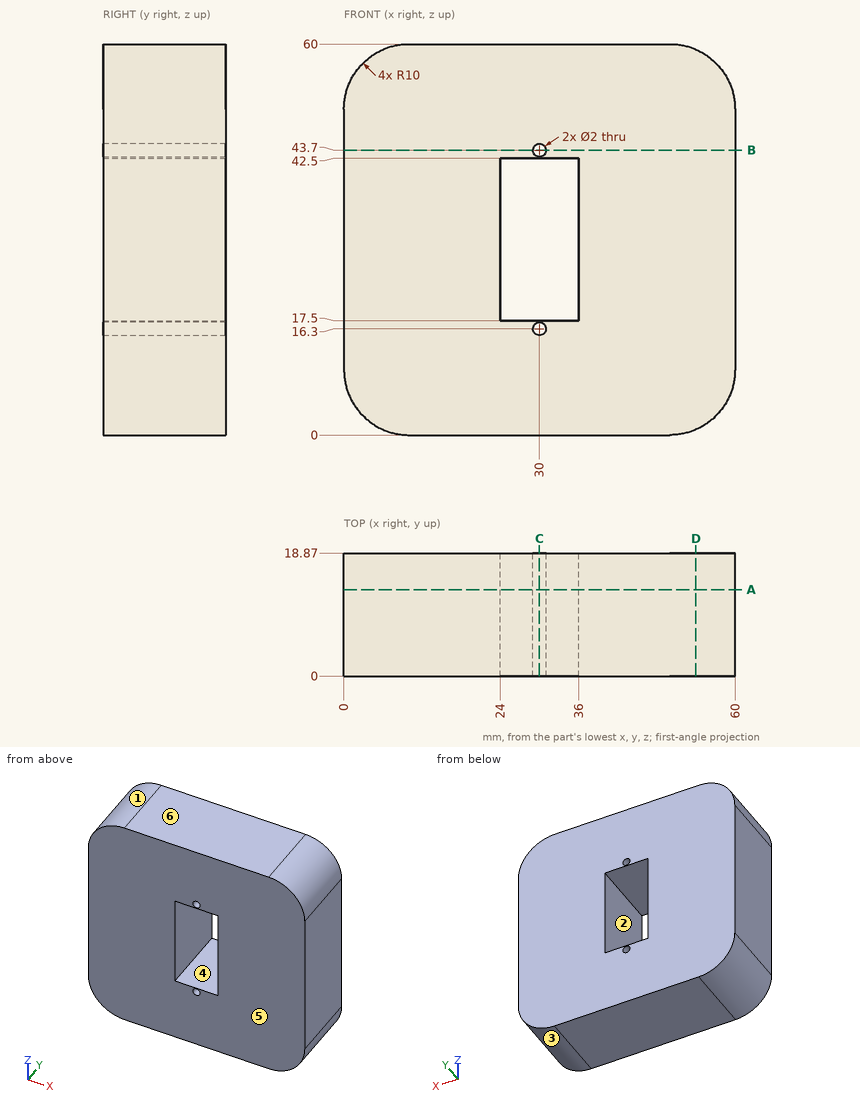
Here's the drawing with two shaded views (mm, measured from the low corner). I have some questions. A direction names the side the tool comes from. Coordinates: 2 decimals unless noted, no trailing zeros. Order: outer loops, then holes, each group sorted by start corner. A loop starts at its lowest first (then second) coordinate and runs counter-clockwise, first axis right, second up.
Item 1: If we section it at D-D on x = 54: List the corners of the cut face in (y, z) for me, plus the area to 3 significant figures.
Result sheet:
outline: (0, 0.83) - (18.87, 0.83) - (18.87, 59.17) - (0, 59.17) - close
area: 1,100 mm2
Item 2: If we section it at B-B on z = 43.7: List the corners of the cut face in (x, y) for me.
Result sheet:
outline: (0, 0) - (29, 0) - (29, 18.87) - (0, 18.87) - close; (31, 0) - (60, 0) - (60, 18.87) - (31, 18.87) - close
Item 3: I need wall thicknesses on line 1 (X direction, y = 5, z = 16.3); line 2 (Z direction, x = 35, y = 11.5); line 3 (X direction, y = 5.75, z = 23). Which ranges of each line are inside material? Lowest first, please.
Result sheet:
line 1: x = 0 to 29, 31 to 60
line 2: z = 0 to 17.5, 42.5 to 60
line 3: x = 0 to 24, 36 to 60
Item 4: If we section it at A-A on y = 13.25: List the corners of the cut face in (x, z) for me.
Result sheet:
outline: (0, 10) arc R10 ccw to (10, 0) - (50, 0) arc R10 ccw to (60, 10) - (60, 50) arc R10 ccw to (50, 60) - (10, 60) arc R10 ccw to (0, 50) - close; hole (24, 17.5) - (36, 17.5) - (36, 42.5) - (24, 42.5) - close; hole circle Ø2 at (30, 16.3); hole circle Ø2 at (30, 43.7)
Item 5: For the marked faces 1 and 2, which set-ups out of +Z, -Z, +X, -X, +Y, -Y let a thin tool reach every point of the face, with its end or its side?
Result sheet:
face 1: +Z, -X, +Y, -Y
face 2: +Y, -Y
Item 6: If we mould it in two halves opening along Z, with no side actions, what happens to the marked faces 3, 4, 5 and 6? For each: +Z half, -Z half, draft (parallel to the pull), parting line (faces both ways), or undercut.
Result sheet:
face 3: -Z half
face 4: undercut
face 5: draft
face 6: +Z half
Item 7: If we section it at C-C on x = 30: List the corners of the cut face in (y, z) for me.
Result sheet:
outline: (0, 0) - (18.87, 0) - (18.87, 15.3) - (0, 15.3) - close; (0, 17.3) - (18.87, 17.3) - (18.87, 17.5) - (0, 17.5) - close; (0, 42.5) - (18.87, 42.5) - (18.87, 42.7) - (0, 42.7) - close; (0, 44.7) - (18.87, 44.7) - (18.87, 60) - (0, 60) - close
